from build123d import *

# Parameters (mm, degrees)
F0_W      = 65.254434
F0_H      = 107.229896
F1_DEPTH  = 7.8625
F2_R      = 5.868431
F3_DEPTH  = 60.29137
F4_DEPTH  = 65.80453
F5_R      = 2.54
F9_DEPTH  = 14.36904
F10_R     = 5.08
F11_R     = 3.805573
F12_DEPTH = 5.85052


with BuildPart() as f1:
    # F0 (on Front) → F1 (new body, symmetric)
    with BuildSketch(Plane.XZ):
        Rectangle(F0_W, F0_H)
    extrude(amount=F1_DEPTH, both=True)

    # F2 (on face) → F3 (cut)
    with BuildSketch(Plane.XZ.offset(7.8625)):
        with BuildLine():
            Line((15.397114, 42.658772), (-15.397114, 42.658772))
            ThreePointArc((-15.397114, 42.658772), (-21.854338, 36.201548), (-15.397114, 29.744324))
            Line((-15.397114, 29.744324), (15.397114, 29.744324))
            ThreePointArc((15.397114, 29.744324), (21.854338, 36.201548), (15.397114, 42.658772))
        make_face()
        with Locations((-20.712784, -40.050827)):
            Circle(F2_R)
    extrude(amount=-F3_DEPTH, mode=Mode.SUBTRACT)

    # F2 (on face) → F4 (cut)
    with BuildSketch(Plane.XZ.offset(7.8625)):
        with BuildLine():
            Line((15.397114, 42.658772), (-15.397114, 42.658772))
            ThreePointArc((-15.397114, 42.658772), (-21.854338, 36.201548), (-15.397114, 29.744324))
            Line((-15.397114, 29.744324), (15.397114, 29.744324))
            ThreePointArc((15.397114, 29.744324), (21.854338, 36.201548), (15.397114, 42.658772))
        make_face()
        with Locations((-20.712784, -40.050827)):
            Circle(F2_R)
    extrude(amount=-F4_DEPTH, mode=Mode.SUBTRACT)

    # F5
    f5_edges = [f1.edges().sort_by_distance(p)[0] for p in [
        (-32.627217, 0, 53.614948),
        (32.627217, 0, 53.614948),
        (32.627217, 0, -53.614948),
        (-32.627217, 0, -53.614948),
        (-32.627217, -7.8625, 0),
        (0, -7.8625, 53.614948),
        (32.627217, -7.8625, 0),
        (0, -7.8625, -53.614948),
    ]]
    fillet(f5_edges, radius=F5_R)

    # F8 (on face) → F9 (join, symmetric)
    with BuildSketch(Plane(origin=(4.31292, 0, -3.978198), x_dir=(0, 1, 0), z_dir=(0.735055, 0, -0.678008))):
        Polygon((-6.416242, -3.535902), (-6.259087, 0), (-23.359215, 8.847466), (-23.359215, 5.644804), align=None)
    extrude(amount=F9_DEPTH, both=True)

    # F10
    f10_edges = [f1.edges().sort_by_distance(p)[0] for p in [
        (-1.336175, -23.359215, 11.090429),
        (19.787886, -23.359215, -8.394213),
    ]]
    fillet(f10_edges, radius=F10_R)

    # F11 (on face) → F12 (cut)
    with BuildSketch(Plane(origin=(-3.675446, -2.937391, -3.984694), x_dir=(0.802896, -0.353719, -0.479834), z_dir=(-0.596119, -0.476414, -0.646276))):
        with Locations((12.278191, 13.279027)):
            Circle(F11_R)
    extrude(amount=-F12_DEPTH, mode=Mode.SUBTRACT)


solid = f1.part
Geometry: final body of the model. Coordinates: model frame, mm. A direction names the side the tool comes from. Give positions to 0.01 mm unless a question says otherwise; leave off trailing zeros. Order: outer loops, then holes, each group sorted by start corner. A loop starts at its lowest first (then second) coordinate and runs counter-clockwise, first axis right, second up. Notation, with made-up numbers: (26, -35) -> (57, -35) arc R24 cw to (57, -17) -> close; hole circle Ø1 at (13, -27.5). An arc over 180 degrees is marked (long way). Put each result on its own line as item: value.
Q1. Reachability of faces 4 (the face through (31.9, -7.1, 0.7)), 5 (the face through (0, 0, 29.744)), 6 (the face through (16.093, -13.144, -12.4)) from +Z, -Z, +X, -X, +Y, -Y: full face, straight path, thin tool, end or side. Return the list, or none.
Here are the results:
face 4: +Z, -Z, +X, -Y
face 5: +Y, -Y
face 6: -Z, +X, -Y
Q2. Material intervals for L1, parallel to Z at x = 15.5, y = 0.5; L2, parallel to Y at x = -21, z = 16; L3, parallel to X at y = -5.5, z = -29, sorted ascending.
Here are the results:
L1: z = -53.61 to 29.75, 42.66 to 53.61
L2: y = -7.86 to 7.86
L3: x = -32.62 to 32.62
Q3. Pin query (flat end, axial travel): pin 1 (10 mm diameter, centred on x = -1, y = -17.5, fed in from -Z); pin 2 (2 mm diameter, centred on x = -2, y = -7.5, fed in from -Z); pin 3 (10 mm diameter, centred on y = -17.5, z = -9.5, fed in from -X). Return the tip coordinate at first contact, or that it passes through.
Here are the results:
pin 1: stops at z = -1.62
pin 2: stops at z = -53.33
pin 3: stops at x = 7.21
Q4. Draft query along X for faces 1 (the face through (-0.784, -21.832, 9.552)), 2 (the face through (0, 7.862, 1)), 3 (the face through (21.853, -0.11, 36.06)). Return one class per face: released by +X, released by -X, zero draft, split by the parting line, or undercut.
Here are the results:
face 1: released by -X
face 2: zero draft
face 3: undercut
Q5. Section C-C, the plane z = 32. Return loops of the section in (x, y), then the cut area to 3 significant figures.
Here are the results:
outline: (-32.63, -5.32) arc R2.54 ccw to (-30.09, -7.86) -> (-20.3, -7.86) -> (-20.3, 7.86) -> (-32.63, 7.86) -> close; (20.3, -7.86) -> (30.09, -7.86) arc R2.54 ccw to (32.63, -5.32) -> (32.63, 7.86) -> (20.3, 7.86) -> close
area: 385 mm^2
Q6. Section B-B, the plane y = -1. Return loops of the section in (x, z), then the cut area to 3 significant figures.
Here are the results:
outline: (-32.63, -51.07) arc R2.54 ccw to (-30.09, -53.61) -> (30.09, -53.61) arc R2.54 ccw to (32.63, -51.07) -> (32.63, 51.07) arc R2.54 ccw to (30.09, 53.61) -> (-30.09, 53.61) arc R2.54 ccw to (-32.63, 51.07) -> close; hole circle Ø11.74 at (-20.71, -40.05); hole (-15.4, 29.74) -> (15.4, 29.74) arc R6.46 ccw to (15.4, 42.66) -> (-15.4, 42.66) arc R6.46 ccw to start
area: 6,350 mm^2
Q7. Section A-A, the plane x = -13.5. Return loops of the section in (y, z).
Here are the results:
outline: (-7.86, -51.07) arc R2.54 ccw to (-5.32, -53.61) -> (7.86, -53.61) -> (7.86, 29.74) -> (-7.86, 29.74) -> close; (-7.86, 42.66) -> (7.86, 42.66) -> (7.86, 53.61) -> (-5.32, 53.61) arc R2.54 ccw to (-7.86, 51.07) -> close
Q8. Section D-D, the plane z = -27. Return loops of the section in (x, y).
Here are the results:
outline: (-32.63, -5.32) arc R2.54 ccw to (-30.09, -7.86) -> (30.09, -7.86) arc R2.54 ccw to (32.63, -5.32) -> (32.63, 7.86) -> (-32.63, 7.86) -> close
